Work out the finished part from the listing and answer in its coordinate system (mm). Coordinates: 2 decimals unless noted, no trailing zeros. Write each loop counter-clockwise with the first axis right and the second up, starting at its lowest first coordinate (ties: lowest second). Pieces come first, ordered by that corner, then holes. Notation, with made-up numbers: (51.5, 17.25) - (107.5, 17.25) arc R17 ccw to (107.5, 33.25) - close; hole circle Ø10 at (-4, 55.25). An arc over 180 degrees is marked (long way). One line per item, written item: value.
```python
from build123d import *

# Parameters (mm, degrees)
SKETCH1_R           = 6.35
BOSS_EXTRUDE1_DEPTH = 9.652
FILLET1_R           = 2.54


with BuildPart() as part:
    # Sketch1 → Boss-Extrude1 (new body)
    with BuildSketch(Plane(origin=(0, 0, 0), x_dir=(1, 0, 0), z_dir=(0, 1, 0))):
        with BuildLine():
            ThreePointArc((-10.16, 30.080506977), (0, 22.86), (10.16, 30.080506977))
            ThreePointArc((10.16, 30.080506977), (15.875, 27.49630657), (20.970483201, 23.839071591))
            ThreePointArc((20.970483201, 23.839071591), (19.797340731, 11.43), (31.130483201, 6.241435386))
            ThreePointArc((31.130483201, 6.241435386), (31.75, 0), (31.130483201, -6.241435386))
            ThreePointArc((31.130483201, -6.241435386), (19.797340731, -11.43), (20.970483201, -23.839071591))
            ThreePointArc((20.970483201, -23.839071591), (15.875, -27.49630657), (10.16, -30.080506977))
            ThreePointArc((10.16, -30.080506977), (0, -22.86), (-10.16, -30.080506977))
            ThreePointArc((-10.16, -30.080506977), (-15.875, -27.49630657), (-20.970483201, -23.839071591))
            ThreePointArc((-20.970483201, -23.839071591), (-19.797340731, -11.43), (-31.130483201, -6.241435386))
            ThreePointArc((-31.130483201, -6.241435386), (-31.75, 0), (-31.130483201, 6.241435386))
            ThreePointArc((-31.130483201, 6.241435386), (-19.797340731, 11.43), (-20.970483201, 23.839071591))
            ThreePointArc((-20.970483201, 23.839071591), (-15.875, 27.49630657), (-10.16, 30.080506977))
        make_face()
        with Locations(Location((0, 0, 0), (0, 0, 270))):
            Circle(SKETCH1_R, mode=Mode.SUBTRACT)
    extrude(amount=BOSS_EXTRUDE1_DEPTH)

    # Fillet1
    fillet1_edges = [part.edges().sort_by_distance(p)[0] for p in [
        (-10.16, 4.826, -30.080506977),
        (10.16, 4.826, -30.080506977),
        (20.970483201, 4.826, -23.839071591),
        (31.130483201, 4.826, -6.241435386),
        (31.130483201, 4.826, 6.241435386),
        (20.970483201, 4.826, 23.839071591),
        (10.16, 4.826, 30.080506977),
        (-10.16, 4.826, 30.080506977),
        (-20.970483201, 4.826, 23.839071591),
        (-31.130483201, 4.826, 6.241435386),
        (-31.130483201, 4.826, -6.241435386),
        (-20.970483201, 4.826, -23.839071591),
    ]]
    fillet(fillet1_edges, radius=FILLET1_R)


solid = part.part
```
Item 1: Section A-A, the plane x = 0 is taken. Determine the outline of the cut face in (y, z).
Evaluation:
outline: (0, -22.86) - (9.65, -22.86) - (9.65, -6.35) - (0, -6.35) - close; (0, 6.35) - (9.65, 6.35) - (9.65, 22.86) - (0, 22.86) - close
Item 2: Consider probe 1 along X at (y, z) = (4.25, 0); probe 2 along X at (y, z) = (9, -26); probe 3 along X at (y, z) = (1.5, 13). Determine where each line is inside the solid, lowest interval first.
Evaluation:
probe 1: x = -31.75 to -6.35, 6.35 to 31.75
probe 2: x = -18.22 to -7.6, 7.6 to 18.22
probe 3: x = -19.05 to 19.05
Item 3: Given pin 1 (8 mm diameter, centred on x = -2.5, z = -20.5, fed in from -Y); pin 2 (1.5 mm diameter, centred on y = 7, z = -20.5, fed in from +X); pin 3 (2 mm diameter, centred on x = -0.5, y = 5.5, fed in from -Z); pin 4 (2 mm diameter, centred on y = 6, z = 12, fed in from +X), each flat-ended and moving along its own axis, determine where each tip first touches the part or whether it passes through.
Evaluation:
pin 1: stops at y = 0
pin 2: stops at x = 19.32
pin 3: stops at z = -22.97
pin 4: stops at x = 20.06
Item 4: Determine the mould class of faces 1 (the face through (-3.86, 4.76, -5.04)), 2 (the face through (-15.92, 4.76, -27.47)), 3 (the face through (19.877, 4.758, 11.295)), 4 (the face through (-7, 9.652, 0)) for opening direction Z: +Z half, -Z half, draft (parallel to the pull), parting line (faces both ways), or undercut.
Evaluation:
face 1: undercut
face 2: -Z half
face 3: undercut
face 4: draft
Item 5: Section C-C, the plane x = -23 is taken. Determine the outline of the cut face in (y, z), then the cut area to 3 significant figures.
Evaluation:
outline: (0, -7.96) - (9.65, -7.96) - (9.65, 7.96) - (0, 7.96) - close
area: 154 mm2
Item 6: Section D-D, the plane z = 19 is taken. Determine the outline of the cut face in (x, y), then the cut area to 3 significant figures.
Evaluation:
outline: (-18.58, 0) - (18.58, 0) - (18.58, 9.65) - (-18.58, 9.65) - close
area: 359 mm2
Item 7: Section B-B, the plane z = 0 is taken. Determine the outline of the cut face in (x, y).
Evaluation:
outline: (-31.75, 0) - (-6.35, 0) - (-6.35, 9.65) - (-31.75, 9.65) - close; (6.35, 0) - (31.75, 0) - (31.75, 9.65) - (6.35, 9.65) - close
